Geometry check sheet. Reference: the model listing, model coordinates, mm. A direction names the side the tool comes from. Give positions to 0.01 mm unless a question says otherwise; leave off trailing zeros. Write each loop counter-clockwise with the first axis right and the second up, starting at its lowest first coordinate (ties: lowest second). Pieces come first, ordered by that corner, then holes. Notation, with made-up numbers: (59.25, 1.25) -> (93.25, 1.25) arc R34 ccw to (93.25, 38.25) -> close; hole circle Ø2 at (82.5, 55.5). An arc over 180 degrees is marked (long way). One line per item, written item: value.
from build123d import *

# Parameters (mm, degrees)
F0_R          = 9.525
F1_DEPTH      = 6.35
F1_DEPTH_BACK = 8.58774
F2_R          = 7.9375
F3_DEPTH      = 123.825
F4_R          = 9.525
F5_DEPTH      = 15.24
F6_DEPTH      = 2.62128


with BuildPart() as f1:
    # F0 (on Right) → F1 (new body, two sides)
    with BuildSketch(Plane.YZ) as f1_sk:
        Circle(F0_R)
    extrude(amount=F1_DEPTH)
    extrude(f1_sk.sketch, amount=-F1_DEPTH_BACK)

    # F2 (on face) → F3 (join)
    with BuildSketch(Plane.YZ.offset(6.35)):
        Circle(F2_R)
    extrude(amount=F3_DEPTH)

    # F4 (on face) → F5 (join)
    with BuildSketch(Plane.YZ.offset(130.175)):
        Circle(F4_R)
    extrude(amount=F5_DEPTH)

    # F6 (add): a face of the model
    f6_faces = [f1.faces().sort_by_distance(p)[0] for p in [
        (145.415, 0, 0),
    ]]
    extrude(f6_faces, amount=F6_DEPTH)


solid = f1.part
1) Scan lines: probe 1 along X at (y, z) = (-6.75, 5) (3 decimals); probe 2 along Y at (x, z) = (140.5, -0.25); probe 3 along Z at (x, y) = (100, -0.5). Record each from-to range of solid material in increasing order.
Verdict:
probe 1: -8.588 to 6.35, 130.175 to 148.036
probe 2: -9.52 to 9.52
probe 3: -7.92 to 7.92
2) Mould release check, pull along X, two halves, no side actions. Record for faces 1 (the flat face through (-8.588, 0, 0)), 2 (the flat face through (130.175, -2, 8)), 3 (the flat face through (6.35, -2, 8)), 4 (the flat face through (148.036, 0, 0)): released by +X, released by -X, zero draft, split by the parting line, or undercut.
Verdict:
face 1: released by -X
face 2: undercut
face 3: undercut
face 4: released by +X
3) Tool access check on faces 5 (the cylindrical face through (-1.014, -7.559, -5.796)), 6 (the cylindrical face through (67.4, -1.72, -7.75)). Record the directions out of +Z, -Z, +X, -X, +Y, -Y that give a thin tool (end or side, any length) a straight path to the whole face; none if there is none.
Verdict:
face 5: +X, -X
face 6: none
4) Sectioned sample at C-C on x = 57. Record the cut outline in (y, z) (1 decimal), plus the area to 3 significant figures.
Verdict:
outline: circle Ø15.9 at (0, 0)
area: 198 mm^2
5) Depth check by flat-ended pin: pin 1 Ø6 at (x, y) = (28.5, 2.5) entering from +Z; pin 2 Ø3 at (x, y) = (40.5, -5.5) entering from +Z; pin 3 Ø1.5 at (x, z) = (29, 7.5) entering from +Y. Enter the tip coordinate at first touch or a pass-through.
Verdict:
pin 1: z = 7.94
pin 2: z = 6.86
pin 3: y = 4.18
